Here's how the part is built. I have some questions about the finished solid (model axes, mm). Round coordinates to 2 decimals unless told otherwise and drop trailing zeros. Loops run counter-clockwise (first coordinate to the right, second up) from the corner with the lowest first, then second, coordinate; pieces in that order, holes last. Notation, with made-up numbers: M -37.5,64.25 L -15.5,64.25 A19 cw -15.5,80.25 Z; hole C -20.5,72.5 d7. An arc over 180 degrees is marked long. Answer as a JSON object with one key per item and string values.
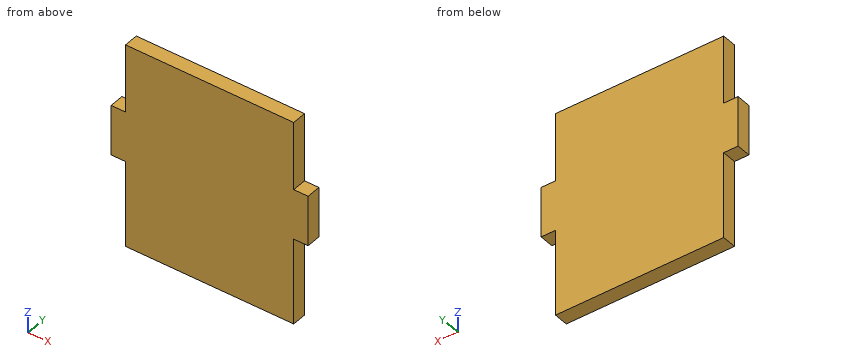
from build123d import *

# Parameters (mm, degrees)
SKETCH1_W           = 23.4
SKETCH1_H           = 28.5
SKETCH1_W_2         = 2
SKETCH1_H_2         = 7
BOSS_EXTRUDE1_DEPTH = 2


with BuildPart() as part:
    # Sketch1 → Boss-Extrude1 (new body)
    with BuildSketch(Plane(origin=(0, 0, 0), x_dir=(1, 0, 0), z_dir=(0, 1, 0))):
        Rectangle(SKETCH1_W, SKETCH1_H)
        with Locations((-12.7, -1.25)):
            Rectangle(SKETCH1_W_2, SKETCH1_H_2)
        with Locations((12.7, -1.25)):
            Rectangle(SKETCH1_W_2, SKETCH1_H_2)
    extrude(amount=BOSS_EXTRUDE1_DEPTH)


solid = part.part
Item 1: For P1, Ø4, axis at x = 7.5, z = -9, coming from the -Y side; P2, Ø0.6, axis at y = 0.5, z = -9, coming from the -X side; P3, Ø1, axis at x = -13, y = 0.5, coming from the +Z side, each with a flat end and sliding along its axis, tell me the tip position at first contact or that it passes through.
Solution:
{"P1": "stops at y = 0", "P2": "stops at x = -11.7", "P3": "stops at z = 4.75"}
Item 2: I want a section at B-B on z = -3. List the corners of the cut face in (x, y) for me, plus the area to 3 significant figures.
Solution:
{"outline": "M -11.7,0 L 11.7,0 L 11.7,2 L -11.7,2 Z", "area": "46.8 mm2"}
Item 3: I want a section at A-A on y = 1.55. List the corners of the cut face in (x, z) for me, plus the area to 3 significant figures.
Solution:
{"outline": "M -13.7,-2.25 L -11.7,-2.25 L -11.7,-14.25 L 11.7,-14.25 L 11.7,-2.25 L 13.7,-2.25 L 13.7,4.75 L 11.7,4.75 L 11.7,14.25 L -11.7,14.25 L -11.7,4.75 L -13.7,4.75 Z", "area": "695 mm2"}
Item 4: If I drill on L1, parallel to X at y = 1.9, z = -4.25; L2, parallel to Z at x = 12.5, y = 1.65, over which ranges is the centre line in solid material (lowest first)? Write a range as from..to.
Solution:
{"L1": "x = -11.7..11.7", "L2": "z = -2.25..4.75"}
